```python
from build123d import *

# Parameters (mm, degrees)
SKETCH1_R           = 7.5
BOSS_EXTRUDE1_DEPTH = 7
SKETCH1_3_R         = 10
SKETCH1_3_R_2       = 7.5
BOSS_EXTRUDE2_DEPTH = 2.2


with BuildPart() as part:
    # Sketch1 → Boss-Extrude1 (new body, symmetric)
    with BuildSketch(Plane(origin=(0, 0, 0), x_dir=(1, 0, 0), z_dir=(0, 1, 0))):
        Circle(SKETCH1_R)
        Polygon((-5.787936449, 0), (-2.893968224, -5.0125), (2.893968224, -5.0125), (5.787936449, 0), (2.893968224, 5.0125), (-2.893968224, 5.0125), align=None, mode=Mode.SUBTRACT)
    extrude(amount=BOSS_EXTRUDE1_DEPTH, both=True)

    # Sketch1_3 → Boss-Extrude2 (add, symmetric)
    with BuildSketch(Plane(origin=(0, 0, 0), x_dir=(1, 0, 0), z_dir=(0, 1, 0))):
        Circle(SKETCH1_3_R)
        Circle(SKETCH1_3_R_2, mode=Mode.SUBTRACT)
        Circle(SKETCH1_3_R_2)
        Polygon((-5.787936449, 0), (-2.893968224, -5.0125), (2.893968224, -5.0125), (5.787936449, 0), (2.893968224, 5.0125), (-2.893968224, 5.0125), align=None, mode=Mode.SUBTRACT)
    extrude(amount=BOSS_EXTRUDE2_DEPTH, both=True)


solid = part.part
```
For this review, take the finished solid that the model builds, in its own axes (mm). A direction names the side the tool comes from. Coordinates: 2 decimals unless noted, no trailing zeros. Loops run counter-clockwise (first coordinate to the right, second up) from the corner with the lowest first, then second, coordinate; pieces in that order, holes last.
1. Add section A-A, the plane y = 0. Give the boundary of the cut face in (x, z).
2. For faces 1 (the flat face through (-4.32, 0.1, -2.54)), 2 (the flat face through (4, 2.2, -7)), 3 (the flat face through (4, -2.2, -7)), list the 3-axis set-ups (+Z, -Z, +X, -X, +Y, -Y) from which the entire face can be reached by the end or side of a thin tool; tool diameter is ignored.
3. Insertion check: P1, Ø4, axis at x = -4, y = 0.5, coming from the +Z side; P2, Ø4, axis at x = 0.5, y = 0, coming from the +Z side; P3, Ø5, axis at y = 2.5, z = 3, coming from the -X side; P4, Ø5, axis at x = -2, y = 5, coming from the -Z side. Each pin has a flat end and moves straight along its axis. Give the tip position at first contact, or say it passes through.
4. Add section D-D, the plane y = 6.25. Give the boundary of the cut face in (x, z), then the cut area to 3 significant figures.
5. Add section B-B, the plane x = 0. Give the boundary of the cut face in (y, z).
6. Mouldability with a two-part tool opening along X and no side actions: class faces 4 (the cylindrical face through (-2.17, 0.03, 9.76)), 5 (the flat face through (5, 7, -2)), 6 (the flat face through (-4.36, 0.1, 2.47)) as +X half, -X half, draft (parallel to the pull), parting line (faces both ways), or undercut.
7. Add section C-C, the plane z = 3.5. Give the boundary of the cut face in (x, y).
8. For line 1 (Z direction, x = 4.5, y = -5.5); line 2 (X direction, y = 1.75, z = 4.5); line 3 (Z direction, x = 2.25, y = 0.25), list the stretches that pass through material, from the lowest coordinate up.
Result:
1. outline: circle Ø20 at (0, 0); hole (-5.79, 0) - (-2.89, -5.01) - (2.89, -5.01) - (5.79, 0) - (2.89, 5.01) - (-2.89, 5.01) - close
2. face 1: +Y, -Y
2. face 2: +Y
2. face 3: -Y
3. P1: stops at z = 9.8
3. P2: stops at z = 10
3. P3: stops at x = -9.99
3. P4: stops at z = -7.5
4. outline: circle Ø15 at (0, 0); hole (-5.79, 0) - (-2.89, -5.01) - (2.89, -5.01) - (5.79, 0) - (2.89, 5.01) - (-2.89, 5.01) - close
4. area: 89.7 mm2
5. outline: (-7, -7.5) - (-2.2, -7.5) - (-2.2, -10) - (2.2, -10) - (2.2, -7.5) - (7, -7.5) - (7, -5.01) - (-7, -5.01) - close; (-7, 5.01) - (7, 5.01) - (7, 7.5) - (2.2, 7.5) - (2.2, 10) - (-2.2, 10) - (-2.2, 7.5) - (-7, 7.5) - close
6. face 4: parting line
6. face 5: draft
6. face 6: undercut
7. outline: (-9.37, -2.2) - (-6.63, -2.2) - (-6.63, -7) - (-3.77, -7) - (-3.77, 7) - (-6.63, 7) - (-6.63, 2.2) - (-9.37, 2.2) - close; (3.77, -7) - (6.63, -7) - (6.63, -2.2) - (9.37, -2.2) - (9.37, 2.2) - (6.63, 2.2) - (6.63, 7) - (3.77, 7) - close
8. line 1: z = -6 to -2.23, 2.23 to 6
8. line 2: x = -8.93 to -3.19, 3.19 to 8.93
8. line 3: z = -9.74 to -5.01, 5.01 to 9.74
